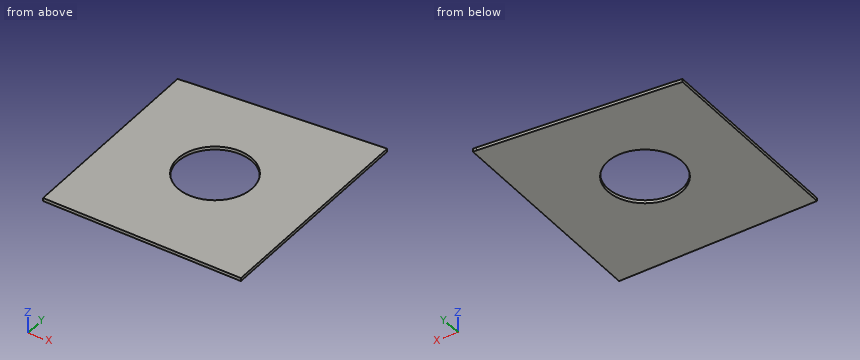
from build123d import *

# Parameters (mm, degrees)
F0_W     = 1215.8472
F0_H     = 1327.15
F1_DEPTH = 19.05
F2_SIZE2 = 104.4195221847
F2_SIZE  = 1193.5206
F3_R     = 228.6
F4_DEPTH = 19.051


with BuildPart() as f1:
    # F0 (on Top) → F1 (new body)
    with BuildSketch(Plane.XY):
        Rectangle(F0_W, F0_H)
    extrude(amount=F1_DEPTH)

    # F2
    f2_edges = [f1.edges().sort_by_distance(p)[0] for p in [
        (-607.9236, 663.575, 9.525),
    ]]
    f2_side = f1.faces().sort_by_distance((0, 663.575, 9.525))[0]
    chamfer(f2_edges, length=F2_SIZE, length2=F2_SIZE2, reference=f2_side)

    # F3 (on face) → F4 (cut, through all)
    with BuildSketch(Plane.XY.offset(19.05)):
        Circle(F3_R)
    extrude(amount=-F4_DEPTH, mode=Mode.SUBTRACT)


solid = f1.part
Model file for the job. Use its own axes, mm. Coordinates: 2 decimals unless noted, no trailing zeros. Order: outer loops, then holes, each group sorted by start corner. A loop starts at its lowest first (then second) coordinate and runs counter-clockwise, first axis right, second up. Notation, with made-up numbers: (24.25, 37.25) -> (70.25, 37.25) arc R23 ccw to (70.25, 76.25) -> close; hole circle Ø7 at (49.25, 88). An arc over 180 degrees is marked (long way). Return JSON: item names as keys, results as strings. Group by question number.
Item 1: Wall check: line 1 along Y through (x, z) = (78.5, 16) (3 decimals); line 2 along X through (y, z) = (-101, 3); line 3 along X through (y, z) = (2.5, 7). Give the ranges that are in metal, low to high. Write a range as [from, to].
Item 2: Saw through at A-A on y = 0. Write the cut outline in (x, z), then the cut area to 3 significant figures.
Item 3: Saw through at D-D on x = -399. Write the cut outline in (y, z) (3 decimals).
Item 4: Saw through at B-B on z = 14. Write the cut outline in (x, y) (3 decimals).
Item 5: Flat gauge pins, fed straight in: P1, Ø4, axis at x = -335.5, y = -464, coming from the -Z side; P2, Ø3, axis at x = -340, z = 13, coming from the +Y side; P3, Ø1.5, axis at x = 5.5, z = 6.5, coming from the +Y side. Where does each tip first touch, or does it go through?
Values found:
{
 "1": {"line 1": "y = [-663.575, -214.699], [214.699, 619.21]", "line 2": "x = [-607.92, -205.08], [205.08, 607.92]", "line 3": "x = [-607.92, -228.59], [228.59, 607.92]"},
 "2": {"outline": "(-607.92, 0) -> (-228.6, 0) -> (-228.6, 19.05) -> (-607.92, 19.05) -> close; (228.6, 0) -> (607.92, 0) -> (607.92, 19.05) -> (228.6, 19.05) -> close", "area": "14,500 mm2"},
 "3": {"outline": "(-663.575, 0) -> (577.434, 0) -> (577.434, 19.05) -> (-663.575, 19.05) -> close"},
 "4": {"outline": "(-607.924, -663.575) -> (607.924, -663.575) -> (607.924, 663.575) -> (585.597, 663.575) -> (-607.924, 559.155) -> close; hole circle Ø457.2 at (0, 0)"},
 "5": {"P1": "stops at z = 0", "P2": "stops at y = 582.73", "P3": "stops at y = 612.89"}
}
